from build123d import *

# Parameters (mm, degrees)
ESBO_O1_R                = 4
RESSALTO_EXTRUS_O2_DEPTH = 10
ESBO_O2_W                = 80
ESBO_O2_H                = 133.630843717
ESBO_O2_R                = 3.25
RESSALTO_EXTRUS_O3_DEPTH = 10


with BuildPart() as part:
    # Esbo_o1 → Ressalto-extrus_o2 (new body)
    with BuildSketch(Plane(origin=(10, 0, 0), x_dir=(0, 0, -1), z_dir=(1, 0, 0))):
        Polygon((0, 0), (76.860522137, 0), (0, -133.630843717), align=None)
        with Locations((45.40940211, -20.909755611)):
            Circle(ESBO_O1_R, mode=Mode.SUBTRACT)
        Polygon((10, -10), (10, -96.187822441), (29.441560186, -62.386437561), (29.441560186, -10), align=None, mode=Mode.SUBTRACT)
    extrude(amount=RESSALTO_EXTRUS_O2_DEPTH)


with BuildPart() as body_2:
    # Espelhar2: mirrored copy
    add(part.part.mirror(Plane(origin=(0, 0, 0), x_dir=(0, 0, 1), z_dir=(1, 0, 0))))


with BuildPart() as part_1:
    add(part.part)

    add(body_2.part)  # Ressalto-extrus_o3 merges body 2
    # Esbo_o2 → Ressalto-extrus_o3 (add)
    with BuildSketch(Plane.XY):
        with Locations((0, -66.815421859)):
            Rectangle(ESBO_O2_W, ESBO_O2_H)
        with Locations((-30, -10)):
            Circle(ESBO_O2_R, mode=Mode.SUBTRACT)
        with Locations((30, -10)):
            Circle(ESBO_O2_R, mode=Mode.SUBTRACT)
        with Locations((-30, -123.630843717)):
            Circle(ESBO_O2_R, mode=Mode.SUBTRACT)
        with Locations((30, -123.630843717)):
            Circle(ESBO_O2_R, mode=Mode.SUBTRACT)
    extrude(amount=RESSALTO_EXTRUS_O3_DEPTH)


solid = part_1.part
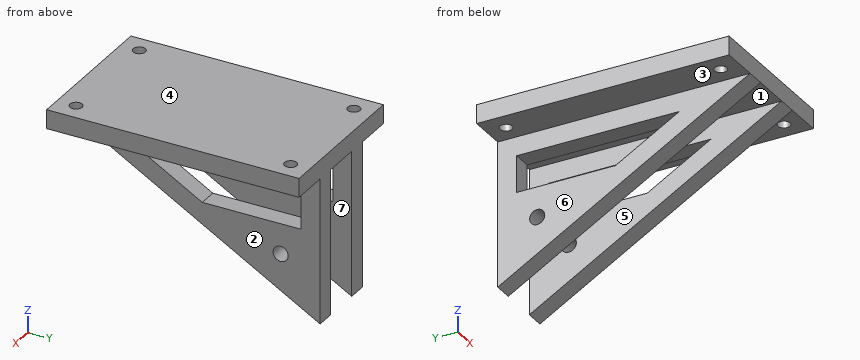
Verification items for the finished model (mm, model axes). Face numbers are marked on the shaded views. A direction names the side the tool comes from. Round coordinates to 2 decimals unless told otherwise and drop trailing zeros. Order: outer loops, then holes, each group sorted by start corner. A loop starts at its lowest first (then second) coordinate and runs counter-clockwise, first axis right, second up.
1. Access from +Z, -Z, +X, -X, +Y, -Y to the whole of each face (thin tool, end or side, straight path). Record for the marked faces 1, 2 and 3.
Final values:
face 1: -Z, +Y, -Y
face 2: -Z, +X, +Y, -Y
face 3: -Z, -X, +Y, -Y
2. Section check B-B on z = -13. Record the cut outline in (x, y), then the cut area to 3 significant figures.
Final values:
outline: (-20, -111.03) - (-10, -111.03) - (-10, -90.97) - (-20, -90.97) - close; (-20, -10) - (-10, -10) - (-10, 0) - (-20, 0) - close; (10, -111.03) - (20, -111.03) - (20, -90.97) - (10, -90.97) - close; (10, -10) - (20, -10) - (20, 0) - (10, 0) - close
area: 601 mm2
3. Release check for a two-part mould opening along X. For the marked faces 4, 5, 6 and 7 record: +X half, -X half, draft (parallel to the pull), parting line (faces both ways), or undercut.
Final values:
face 4: draft
face 5: undercut
face 6: -X half
face 7: undercut
4. Go/stop test with flat-tipped pins: P1, Ø10, axis at x = -26, y = -67.5, coming from the -Z side; P2, Ø8, axis at x = 15, z = -20, coming from the -Y side; P3, Ø5, axis at x = 17, y = -47, coming from the -Z side. Record where each tip stops, or that it passes through.
Final values:
P1: stops at z = 0
P2: stops at y = -105.81
P3: stops at z = -51.27
5. Section check C-C on y = -43. Record the cut outline in (x, z), then the cut area to 3 significant figures.
Final values:
outline: (-40, 0) - (-20, 0) - (-20, -10) - (-10, -10) - (-10, 0) - (10, 0) - (10, -10) - (20, -10) - (20, 0) - (40, 0) - (40, 10) - (-40, 10) - close; (-20, -52.13) - (-10, -52.13) - (-10, -29.44) - (-20, -29.44) - close; (10, -52.13) - (20, -52.13) - (20, -29.44) - (10, -29.44) - close
area: 1,450 mm2
6. Thickness scan on L1, parallel to Y at x = -30, z = 7.5; L2, parallel to X at y = -16, z = -67.5; L3, parallel to Z at x = -1, y = -72. Record the ranges inside material, lowest first.
Final values:
L1: y = -133.63 to -126.88, -120.38 to -13.25, -6.75 to 0
L2: x = -20 to -10, 10 to 20
L3: z = 0 to 10
7. Section check D-D on z = -66. Record the cut outline in (x, y), then the cut area to 3 significant figures.
Final values:
outline: (-20, -18.88) - (-10, -18.88) - (-10, 0) - (-20, 0) - close; (10, -18.88) - (20, -18.88) - (20, 0) - (10, 0) - close
area: 378 mm2
8. Section check A-A on x = -30. Record the cut outline in (y, z), then the cut area to 3 significant figures.
Final values:
outline: (-133.63, 0) - (-126.88, 0) - (-126.88, 10) - (-133.63, 10) - close; (-120.38, 0) - (-13.25, 0) - (-13.25, 10) - (-120.38, 10) - close; (-6.75, 0) - (0, 0) - (0, 10) - (-6.75, 10) - close
area: 1,210 mm2
